from build123d import *

# Parameters (mm, degrees)
M3_CLEARANCE_HOLE1_D     = 3.4
M3_CLEARANCE_HOLE1_DEPTH = 7.5673


with BuildPart() as part:
    # Sketch1 → Revolve1 (revolve)
    with BuildSketch(Plane.XY, mode=Mode.PRIVATE) as revolve1_sk:
        Polygon((5.12, 5), (5.12, 13.8632), (5.5, 13.8632), (14.1, 10.3613), (14.1, 7.5673), (22, 7.5673), (22, 0), (6.75, 0), (6.75, 5), align=None)
    revolve(revolve1_sk.sketch.rotate(Axis((0, 0, 0), (0, 1, 0)), 90), axis=Axis((0, 0, 0), (0, 1, 0)))

    # M3 Clearance Hole1
    with Locations(Plane(origin=(0, 7.5673, 0), x_dir=(1, 0, 0), z_dir=(0, 1, 0))):
        with Locations((0, 19), (16.454482672, 9.5), (16.454482672, -9.5), (0, -19), (-16.454482672, -9.5), (-16.454482672, 9.5), (0, 0)):
            Hole(M3_CLEARANCE_HOLE1_D / 2, depth=M3_CLEARANCE_HOLE1_DEPTH)


solid = part.part
Here's how the part is built. I have some questions about the finished solid (model axes, mm). A direction names the side the tool comes from. Round coordinates to 2 decimals unless told otherwise and drop trailing zeros. Loops run counter-clockwise (first coordinate to the right, second up) from the corner with the lowest first, then second, coordinate; pieces in that order, holes last. Notation, with made-up numbers: M 56.25,73.5 L 61.25,73.5 A14 ccw 61.25,80.5 Z; hole C 52,15 d5. An arc over 180 degrees is marked long. Write each question's results on one line, items separated by ' | '. Start each with the question number.
(1) I want a section at C-C (x = -17). Please give me the cut outline in (y, z), then the cut area to 3 significant figures.
(2) If I drill on probe 1 along X at (y, z) = (9.75, 0); probe 2 along Z at (x, y) = (0.5, 1.75); probe 3 along X at (y, z) = (5.75, 9.5), over which ranges is the centre line in solid material (lowest first)? Write a range as from..to.
(3) Will these pins go through, and if not, where does the flat tip stop? P1, Ø4, axis at x = 1.5, z = -17, coming from the +Y side; P2, Ø12, axis at x = 0, z = 0, coming from the -Y side; P3, Ø1, axis at y = 6, z = -14, coming from the +X side; P4, Ø2, axis at x = 16.45, z = -9.5, coming from the -Y side.
(4) I want a section at D-D (y = 8.5). Please give me the cut outline in (x, z), then the cut area to 3 significant figures.
(5) I want a section at B-B (z = 19). Please give me the cut outline in (x, y).
(6) On a 3-axis mill with a long thin cutter (end or side, diameter ignored), from which of +Z, -Z, +X, -X, +Y, -Y can I reach the whole of each face in a straight line? I mean faces 4 (the flat face through (14.4, 7.567, -0.3)), 5 (the flat face through (-5, 5, -2)), 6 (the cylindrical face through (21.477, 3.731, 4.769)). Say none if no direction works.
(7) I want a section at A-A (y = 3). Please give me the cut outline in (x, z).
(8) Thinking about a two-plate mould opening in X: for faces 1 (the cylindrical face through (18.153, 3.731, -9.575)), 2 (the cylindrical face through (13.765, 8.945, 3.057)), 3 (the flat face through (5, 0, 5)), which applies, pulls with the +X half, pulls with the -X half, needs draft (parallel to the pull), parting line crosses it, or undercut?
Solved:
1) outline: M 0,-13.96 L 7.57,-13.96 L 7.57,-11.11 L 0,-11.11 Z; M 0,-7.89 L 7.57,-7.89 L 7.57,7.89 L 0,7.89 Z; M 0,11.11 L 7.57,11.11 L 7.57,13.96 L 0,13.96 Z | area: 163 mm²
2) probe 1: x = -14.1..-5.12, 5.12..14.1 | probe 2: z = -21.99..-20.62, -17.38..-6.73, 6.73..17.38, 20.62..21.99 | probe 3: x = -19.84..-18.15, -14.75..14.75, 18.15..19.84
3) P1: stops at y = 7.57 | P2: stops at y = 5 | P3: stops at x = 17.37 | P4: passes through
4) outline: C 0,0 d28.2; hole C 0,0 d10.24 | area: 542 mm²
5) outline: M -11.09,0 L -1.7,0 L -1.7,7.57 L -11.09,7.57 Z; M 1.7,0 L 11.09,0 L 11.09,7.57 L 1.7,7.57 Z
6) face 4: +Y | face 5: -Y | face 6: +Y, -Y
7) outline: C 0,0 d44; hole C -16.45,-9.5 d3.4; hole C -16.45,9.5 d3.4; hole C 0,0 d13.5; hole C 0,-19 d3.4; hole C 0,19 d3.4; hole C 16.45,-9.5 d3.4; hole C 16.45,9.5 d3.4
8) face 1: undercut | face 2: parting line crosses it | face 3: needs draft
